The listing builds one solid part. Answer for the finished solid, in the listing's coordinates (mm). A direction names the side the tool comes from. Coordinates: 2 decimals unless noted, no trailing zeros. Order: outer loops, then holes, each group sorted by start corner. A loop starts at its lowest first (then second) coordinate and runs counter-clockwise, first axis right, second up. Notation, with made-up numbers: (69.25, -3.5) -> (98.25, -3.5) arc R19 cw to (98.25, 8.5) -> close; hole circle Ø3 at (49.5, 40.25). An arc over 180 degrees is marked (long way). Write item = value, one per line.
from build123d import *

# Parameters (mm, degrees)
BOSS_EXTRUDE3_DEPTH = 30
BOSS_EXTRUDE4_DEPTH = 4.5
CUT_EXTRUDE3_DEPTH  = 4.5
CUT_EXTRUDE4_DEPTH  = 4.5
SKETCH9_R           = 1.5
CUT_EXTRUDE5_DEPTH  = 4.5
CUT_EXTRUDE6_DEPTH  = 3
SKETCH12_R          = 1.5
CUT_EXTRUDE8_DEPTH  = 50.5
CUT_EXTRUDE9_DEPTH  = 3
SKETCH14_R          = 1.5
CUT_EXTRUDE10_DEPTH = 50.5
CUT_EXTRUDE11_DEPTH = 3


with BuildPart() as part:
    # Sketch1 → Boss-Extrude3 (new body)
    with BuildSketch(Plane.XY):
        Polygon((0, 0), (0, 30), (4.5, 30), (4.5, 4.5), (30, 4.5), (30, 0), align=None)
    extrude(amount=BOSS_EXTRUDE3_DEPTH)

    # Sketch6 → Boss-Extrude4 (add)
    with BuildSketch(Plane(origin=(0, 0, 0), x_dir=(-1, 0, 0), z_dir=(0, 0, -1))):
        with BuildLine():
            Line((0, 0), (0, 30))
            Line((0, 30), (-4.5, 30))
            ThreePointArc((-4.5, 30), (-22.53122292, 22.53122292), (-30, 4.5))
            Line((-30, 4.5), (-30, 0))
            Line((-30, 0), (0, 0))
        make_face()
    extrude(amount=-BOSS_EXTRUDE4_DEPTH)

    # Sketch7 → Cut-Extrude3 (cut)
    with BuildSketch(Plane(origin=(4.5, 0, 0), x_dir=(0, 0, -1), z_dir=(1, 0, 0))):
        with BuildLine():
            Line((-30, 4.5), (-56.330793143, 4.5))
            Line((-56.330793143, 4.5), (-56.330793143, 46.447924187))
            Line((-56.330793143, 46.447924187), (-4.5, 46.447924187))
            Line((-4.5, 46.447924187), (-4.5, 30))
            ThreePointArc((-4.5, 30), (-22.53122292, 22.53122292), (-30, 4.5))
        make_face()
    extrude(amount=-CUT_EXTRUDE3_DEPTH, mode=Mode.SUBTRACT)

    # Sketch8 → Cut-Extrude4 (cut)
    with BuildSketch(Plane(origin=(0, 4.5, 0), x_dir=(1, 0, 0), z_dir=(0, 1, 0))):
        with BuildLine():
            Line((4.5, -30), (4.5, -32.471065144))
            Line((4.5, -32.471065144), (33.329643203, -32.471065144))
            Line((33.329643203, -32.471065144), (33.329643203, -4.5))
            Line((33.329643203, -4.5), (30, -4.5))
            ThreePointArc((30, -4.5), (22.53122292, -22.53122292), (4.5, -30))
        make_face()
    extrude(amount=-CUT_EXTRUDE4_DEPTH, mode=Mode.SUBTRACT)

    # Sketch9 → Cut-Extrude5 (cut)
    with BuildSketch(Plane.XY.offset(4.5)):
        with Locations((16, 16)):
            Circle(SKETCH9_R)
    extrude(amount=-CUT_EXTRUDE5_DEPTH, mode=Mode.SUBTRACT)

    # Sketch10 → Cut-Extrude6 (cut)
    with BuildSketch(Plane.XY.offset(4.5)):
        Polygon((19.464101615, 16), (17.732050808, 19), (14.267949192, 19), (12.535898385, 16), (14.267949192, 13), (17.732050808, 13), align=None)
    extrude(amount=-CUT_EXTRUDE6_DEPTH, mode=Mode.SUBTRACT)

    # Sketch12 → Cut-Extrude8 (cut, through all)
    with BuildSketch(Plane(origin=(0, 4.5, 0), x_dir=(1, 0, 0), z_dir=(0, 1, 0))):
        with Locations(Location((16, -16, 0), (0, 0, 180))):
            Circle(SKETCH12_R)
    extrude(amount=-CUT_EXTRUDE8_DEPTH, mode=Mode.SUBTRACT)

    # Sketch13 → Cut-Extrude9 (cut)
    with BuildSketch(Plane(origin=(0, 4.5, 0), x_dir=(1, 0, 0), z_dir=(0, 1, 0))):
        Polygon((19.464101615, -16), (17.732050808, -13), (14.267949192, -13), (12.535898385, -16), (14.267949192, -19), (17.732050808, -19), align=None)
    extrude(amount=-CUT_EXTRUDE9_DEPTH, mode=Mode.SUBTRACT)

    # Sketch14 → Cut-Extrude10 (cut, through all)
    with BuildSketch(Plane(origin=(4.5, 0, 0), x_dir=(0, 0, -1), z_dir=(1, 0, 0))):
        with Locations(Location((-16, 16, 0), (0, 0, 90))):
            Circle(SKETCH14_R)
    extrude(amount=-CUT_EXTRUDE10_DEPTH, mode=Mode.SUBTRACT)

    # Sketch15 → Cut-Extrude11 (cut)
    with BuildSketch(Plane(origin=(4.5, 0, 0), x_dir=(0, 0, -1), z_dir=(1, 0, 0))):
        Polygon((-19.464101615, 16), (-17.732050808, 13), (-14.267949192, 13), (-12.535898385, 16), (-14.267949192, 19), (-17.732050808, 19), align=None)
    extrude(amount=-CUT_EXTRUDE11_DEPTH, mode=Mode.SUBTRACT)


solid = part.part
Q1. Each of these flat-tipped pins is pushed along its axis until it touches: pin 1 Ø1.5 at (x, z) = (3, 15.5) entering from -Y; pin 2 Ø5 at (x, z) = (9.5, 8) entering from +Y; pin 3 Ø0.9 at (x, y) = (15.5, 2.5) entering from +Z; pin 4 Ø1.8 at (x, y) = (16.5, 16) entering from +Z. Where does it stop, or does it pass through?
The answers:
pin_1 = 0
pin_2 = 4.5
pin_3 = 27.72
pin_4 = through
Q2. Find the intervals of material crossed by line 1 along Z through (x, y) = (8, 20), in increasing order.
The answers:
line_1 = 0 to 4.5
Q3. Section D-D, the plane y = 15 is taken. Give the vertices of the cut face in (x, z).
The answers:
outline = (0, 0) -> (14.88, 0) -> (14.88, 1.5) -> (13.11, 1.5) -> (13.11, 4.5) -> (4.5, 4.5) -> (4.5, 13.11) -> (1.5, 13.11) -> (1.5, 14.88) -> (0, 14.88) -> close; (0, 17.12) -> (1.5, 17.12) -> (1.5, 18.89) -> (4.5, 18.89) -> (4.5, 27.74) -> (0, 27.74) -> close; (17.12, 0) -> (27.74, 0) -> (27.74, 4.5) -> (18.89, 4.5) -> (18.89, 1.5) -> (17.12, 1.5) -> close
Q4. Section A-A, the plane y = 3 is taken. Give the vertices of the cut face in (x, z), plus the area to 3 significant figures.
The answers:
outline = (0, 0) -> (30, 0) -> (30, 4.5) arc R25.5 ccw to (4.5, 30) -> (0, 30) -> close; hole (12.54, 16) -> (14.27, 13) -> (17.73, 13) -> (19.46, 16) -> (17.73, 19) -> (14.27, 19) -> close
area = 729 mm2
Q5. The mould has two halves that part along Z. Classify faces 4 (the face through (2.28, 22.73, 22.33)), 5 (the face through (11, 4.5, 14)), 6 (the face through (3, 17.5, 13.4)): released by +Z, released by -Z, zero draft, split by the parting line, or undercut.
The answers:
face_4 = released by +Z
face_5 = zero draft
face_6 = undercut
Q6. Section C-C, the plane x = 16 is taken. Give the vertices of the cut face in (y, z).
The answers:
outline = (0, 0) -> (14.5, 0) -> (14.5, 1.5) -> (13, 1.5) -> (13, 4.5) -> (4.5, 4.5) -> (4.5, 13) -> (1.5, 13) -> (1.5, 14.5) -> (0, 14.5) -> close; (0, 17.5) -> (1.5, 17.5) -> (1.5, 19) -> (4.5, 19) -> (4.5, 27.26) -> (0, 27.26) -> close; (17.5, 0) -> (27.26, 0) -> (27.26, 4.5) -> (19, 4.5) -> (19, 1.5) -> (17.5, 1.5) -> close
Q7. A tool of negligible diameter and unlimited length cuts with its end or side. For faces 1 (the face through (13.4, 3, 17.5)), 2 (the face through (17.5, 16.7, 1.5)), 3 (the face through (3, 17.5, 18.6)), from which of +Z, -Z, +X, -X, +Y, -Y can it reach the whole face along a straight path? Write none if from no direction.
The answers:
face_1 = +Y
face_2 = +Z
face_3 = +X
